Part model, mm, in its own coordinate system. A direction names the side the tool comes from. Round coordinates to 2 decimals unless told otherwise and drop trailing zeros. Loops run counter-clockwise (first coordinate to the right, second up) from the corner with the lowest first, then second, coordinate; pieces in that order, holes last.
1) Band-saw the part on B-B, the plane y = -3. Write the cut outline in (x, z).
2) Band-saw the part on D-D, the plane x = -5.5. Write the cut outline in (y, z).
3) Mould opens along Y. For faces 1 (the cylindrical face through (-0.247, 18.384, 1.479)), 2 (the flat face through (-0.301, -4.477, 3)), 3 (the cylindrical face through (-2.799, 21.317, 1.479)) say: +Y half, -Y half, draft (parallel to the pull), parting line (faces both ways), or undercut.
4) Probe line 1 (X direction, y = 3, z = 1.65); line 2 (Y direction, x = -14.5, z = 2.6); line 3 (X direction, y = 9.5, z = 1.1). List the from-to ranges inside material, lowest first.
5) 3-axis set-ups, long thin cutter, end or side, ignore diameter. For faces 4 (the cylindrical face through (15.166, 6.564, 1.479)), 5 (the flat face through (0, 0, 1.8)): which of +Z, -Z, +X, -X, +Y, -Y reach the whole face in a straight line?
6) Band-saw the part on A-A, the plane x = 0. Write the cut outline in (y, z).
7) Band-saw the part on C-C, the plane y = -16.5. Write the cut outline in (x, z).
8) Drop flat-ended pins along their axis: P1, Ø3, axis at x = 0, y = 16.5, coming from the +Z side; P2, Ø1.5, axis at y = -11.5, z = 2, coming from the -X side; P3, Ø2.5, axis at x = -1.5, y = -1, coming from the +Z side. Give the stop position or say it passes through.
from build123d import *

# Parameters (mm, degrees)
SKETCH_1_R               = 21.5
EXTRUDE_1_DEPTH          = 3
CUT_EXTRUDE_1_DEPTH      = 31.553232235
CUT_EXTRUDE_1_DEPTH_BACK = 31.553232235
SKETCH_2_R               = 1.4
CUT_EXTRUDE_2_DEPTH      = 31.553232235
CUT_EXTRUDE_2_DEPTH_BACK = 31.553232235
SKETCH_3_R               = 1.9
CUT_EXTRUDE_3_DEPTH      = 31.553232235
CUT_EXTRUDE_3_DEPTH_BACK = 1.2
SKETCH_4_R               = 4.1


with BuildPart() as part:
    # ｽｹｯﾁ1 → ﾎﾞｽ - 押し出し1 (new body)
    with BuildSketch(Plane.XY):
        Circle(SKETCH_1_R)
    extrude(amount=EXTRUDE_1_DEPTH)

    # ｽｹｯﾁ2 → ｶｯﾄ - 押し出し1 (cut, two sides: drawn at the far end of the back side and taken through both)
    with BuildSketch(Plane.XY.offset(-CUT_EXTRUDE_1_DEPTH_BACK)):
        with Locations((0, 6)):
            Circle(SKETCH_2_R)
        with Locations((5.196152423, 3)):
            Circle(SKETCH_2_R)
        with Locations((5.196152423, -3)):
            Circle(SKETCH_2_R)
        with Locations((0, -6)):
            Circle(SKETCH_2_R)
        with Locations((-5.196152423, -3)):
            Circle(SKETCH_2_R)
        with Locations((-5.196152423, 3)):
            Circle(SKETCH_2_R)
    extrude(amount=CUT_EXTRUDE_1_DEPTH + CUT_EXTRUDE_1_DEPTH_BACK, mode=Mode.SUBTRACT)

    # ｽｹｯﾁ3 → ｶｯﾄ - 押し出し2 (cut, two sides: drawn at the far end of the back side and taken through both)
    with BuildSketch(Plane.XY.offset(3).offset(-CUT_EXTRUDE_2_DEPTH_BACK)):
        with Locations((0, 16.5)):
            Circle(SKETCH_3_R)
        with Locations((14.289419162, 8.25)):
            Circle(SKETCH_3_R)
        with Locations((14.289419162, -8.25)):
            Circle(SKETCH_3_R)
        with Locations((0, -16.5)):
            Circle(SKETCH_3_R)
        with Locations((-14.289419162, -8.25)):
            Circle(SKETCH_3_R)
        with Locations((-14.289419162, 8.25)):
            Circle(SKETCH_3_R)
    extrude(amount=CUT_EXTRUDE_2_DEPTH + CUT_EXTRUDE_2_DEPTH_BACK, mode=Mode.SUBTRACT)

    # ｽｹｯﾁ4 → ｶｯﾄ - 押し出し3 (cut, two sides: drawn at the far end of the back side and taken through both)
    with BuildSketch(Plane.XY.offset(3).offset(-CUT_EXTRUDE_3_DEPTH_BACK)):
        with Locations(Location((0, 0, 0), (0, 0, 180))):
            Circle(SKETCH_4_R)
    extrude(amount=CUT_EXTRUDE_3_DEPTH + CUT_EXTRUDE_3_DEPTH_BACK, mode=Mode.SUBTRACT)


solid = part.part
Reported:
1. outline: (-21.29, 0) - (-6.6, 0) - (-6.6, 3) - (-21.29, 3) - close; (-3.8, 0) - (3.8, 0) - (3.8, 3) - (2.79, 3) - (2.79, 1.8) - (-2.79, 1.8) - (-2.79, 3) - (-3.8, 3) - close; (6.6, 0) - (21.29, 0) - (21.29, 3) - (6.6, 3) - close
2. outline: (-20.78, 0) - (-4.37, 0) - (-4.37, 3) - (-20.78, 3) - close; (-1.63, 0) - (1.63, 0) - (1.63, 3) - (-1.63, 3) - close; (4.37, 0) - (20.78, 0) - (20.78, 3) - (4.37, 3) - close
3. face 1: undercut
3. face 2: draft
3. face 3: parting line
4. line 1: x = -21.29 to -6.6, -3.8 to 3.8, 6.6 to 21.29
4. line 2: y = -15.87 to -10.14, -6.36 to 6.36, 10.14 to 15.87
4. line 3: x = -19.29 to -15.72, -12.86 to 12.86, 15.72 to 19.29
5. face 4: +Z, -Z
5. face 5: +Z
6. outline: (-21.5, 0) - (-18.4, 0) - (-18.4, 3) - (-21.5, 3) - close; (-14.6, 0) - (-7.4, 0) - (-7.4, 3) - (-14.6, 3) - close; (-4.6, 0) - (4.6, 0) - (4.6, 3) - (4.1, 3) - (4.1, 1.8) - (-4.1, 1.8) - (-4.1, 3) - (-4.6, 3) - close; (7.4, 0) - (14.6, 0) - (14.6, 3) - (7.4, 3) - close; (18.4, 0) - (21.5, 0) - (21.5, 3) - (18.4, 3) - close
7. outline: (-13.78, 0) - (-1.9, 0) - (-1.9, 3) - (-13.78, 3) - close; (1.9, 0) - (13.78, 0) - (13.78, 3) - (1.9, 3) - close
8. P1: passes through
8. P2: stops at x = -18.62
8. P3: stops at z = 1.8
